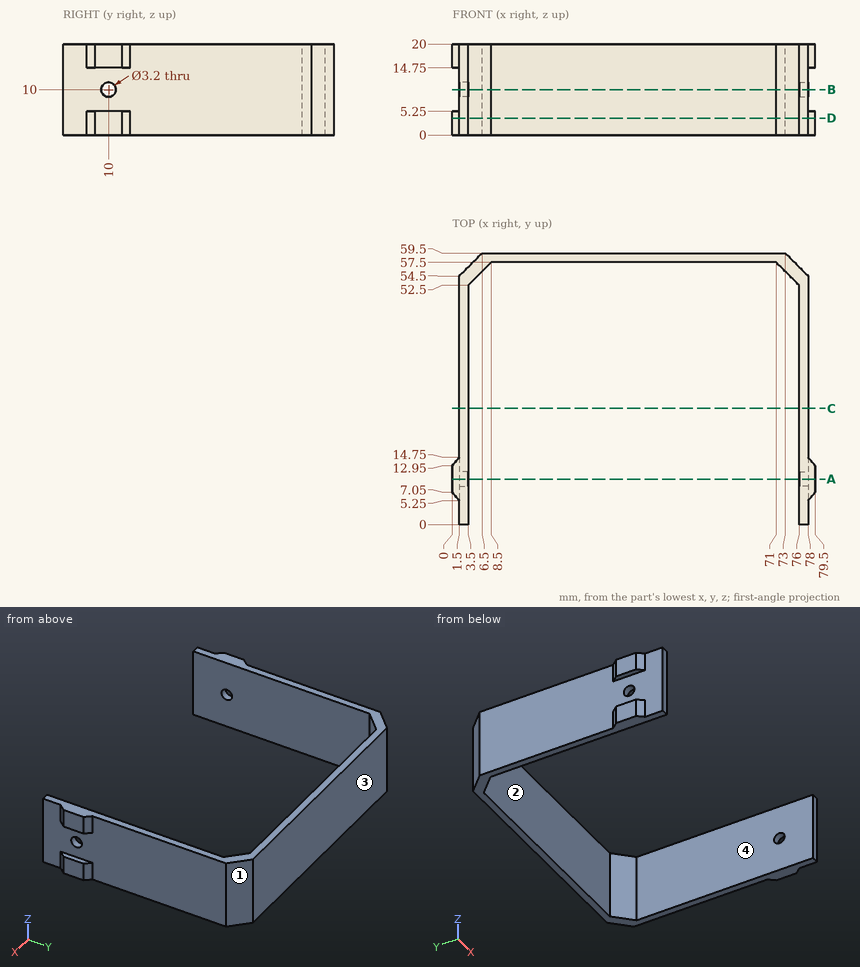
The drawing under review shows one solid part. Ordinate dimensions are in mm from its lowest x, y, z. Round coordinates to 2 decimals unless told otherwise and drop trailing zeros. Write each loop counter-clockwise with the first axis right and the second up, starting at its lowest first coordinate (ties: lowest second). Pieces come first, ordered by that corner, then holes. Notation, with made-up numbers: (-7.75, 2) - (11.25, 2) arc R26 cw to (11.25, 16) - close; hole circle Ø8 at (47, 65). An arc over 180 degrees is marked (long way). Put each result on its own line as item: value.
Q1. Insertion check: pin 1 Ø1.5 at (y, z) = (17.5, 12.5) entering from +X; pin 2 Ø3 at (y, z) = (10, 10) entering from -X; pin 3 Ø6 at (x, z) = (40, 7) entering from -Y; pin 4 Ø8 at (y, z) = (6.5, 9.5) entering from -X. Each pin has a flat end and moves straight along its axis. Give the tip position at first contact, or say it passes through.
Solved:
pin 1: stops at x = 78
pin 2: passes through
pin 3: stops at y = 57.5
pin 4: stops at x = 1.5
Q2. Wall thickness on probe 1 along X at (y, z) = (8, 12.25); probe 2 along Z at (x, y) = (77.3, 10); probe 3 along X at (y, z) = (8, 15.75): over which ranges is each line inside the solid? List them lowest first.
Solved:
probe 1: x = 1.5 to 3.5, 76 to 78
probe 2: z = 0 to 8.4, 11.6 to 20
probe 3: x = 0 to 3.5, 76 to 79.5
Q3. We need section B-B (z = 10). Give the boundary of the cut face in (x, y), and give its area (3 significant figures).
Solved:
outline: (1.5, 0) - (3.5, 0) - (3.5, 8.4) - (1.5, 8.4) - close; (1.5, 11.6) - (3.5, 11.6) - (3.5, 52.5) - (8.5, 57.5) - (71, 57.5) - (76, 52.5) - (76, 11.6) - (78, 11.6) - (78, 54.5) - (73, 59.5) - (6.5, 59.5) - (1.5, 54.5) - close; (76, 0) - (78, 0) - (78, 8.4) - (76, 8.4) - close
area: 370 mm2
Q4. We need section C-C (y = 25.5). Give the boundary of the cut face in (x, z).
Solved:
outline: (1.5, 0) - (3.5, 0) - (3.5, 20) - (1.5, 20) - close; (76, 0) - (78, 0) - (78, 20) - (76, 20) - close
Q5. We need section A-A (y = 10). Give the boundary of the cut face in (x, z).
Solved:
outline: (0, 0) - (3.5, 0) - (3.5, 8.4) - (1.5, 8.4) - (1.5, 5.25) - (0, 5.25) - close; (0, 14.75) - (1.5, 14.75) - (1.5, 11.6) - (3.5, 11.6) - (3.5, 20) - (0, 20) - close; (76, 0) - (79.5, 0) - (79.5, 5.25) - (78, 5.25) - (78, 8.4) - (76, 8.4) - close; (76, 11.6) - (78, 11.6) - (78, 14.75) - (79.5, 14.75) - (79.5, 20) - (76, 20) - close
Q6. We need section D-D (z = 3.75). Give the boundary of the cut face in (x, y), and give its area (3 significant figures).
Solved:
outline: (0, 7.05) - (1.5, 5.25) - (1.5, 0) - (3.5, 0) - (3.5, 52.5) - (8.5, 57.5) - (71, 57.5) - (76, 52.5) - (76, 0) - (78, 0) - (78, 5.25) - (79.5, 7.05) - (79.5, 12.95) - (78, 14.75) - (78, 54.5) - (73, 59.5) - (6.5, 59.5) - (1.5, 54.5) - (1.5, 14.75) - (0, 12.95) - close
area: 406 mm2
Q7. Mouldability with a two-part tool opening along X and no side actions: class the marked faces 1, 2, 3 and 4 as released by +X, released by -X, zero draft, split by the parting line, or undercut.
Solved:
face 1: released by +X
face 2: undercut
face 3: zero draft
face 4: undercut
